Can you work these out from the model? Positions are in its coordinate system, mm. A direction names the side the tool comes from. Coordinates: 2 decimals unless noted, no trailing zeros. Order: outer loops, then holes, each group sorted by start corner. A loop starts at its lowest first (then second) coordinate and runs counter-clockwise, first axis right, second up. Notation, with made-up numbers: (80.25, 44.5) -> (86.25, 44.5) arc R17 cw to (86.25, 49.5) -> close; hole circle Ø11 at (67, 46.25). An arc over 180 degrees is marked (long way). Answer as a JSON object with one key per item and string values. Group by question number.
(1) I want a section at B-B, the plane z = -24.5. List the corners of the cut face in (x, y) for me.
(2) I need wall thicknesses on line 1 (X direction, y = 1, z = -24.5); line 2 (Z direction, x = -52.5, y = 2.45); line 3 (X direction, y = 1.9, z = -18). Which ranges of each line are inside material? Lowest first, please.
(3) I want a section at C-C, the plane y = 1.75. State how many separate pieces and enclosed holes the cut face has, plus the area to 3 significant figures.
(4) I want a section at A-A, the plane x = 52.5. List the corners of the cut face in (y, z) for me, plus the area to 3 significant figures.
(5) For pin 1 (5 mm diameter, centred on x = 30.5, y = 8, fed in from +Z); pin 2 (1.8 mm diameter, centred on x = 18, y = 7.5, fed in from +Z); pin 3 (1.3 mm diameter, centred on x = -12, y = 8, fed in from -Z); pin 4 (1 mm diameter, centred on x = 4, z = -8, fed in from +Y), each with a flat end and sliding along its axis, tell me the tip position at first contact or that it passes through.
(6) If we mould it in two halves opening along Z, with no side actions, what happens to faces 1 (the flat face through (15, 5, 18)), 2 (the flat face through (12, 5, 3)), 3 (the cylindrical face through (54.2, 1.48, -28.07))? For each: pulls with the +Z half, pulls with the -Z half, needs draft (parallel to the pull), parting line crosses it, or undercut.
(7) Which directions (+Z, -Z, +X, -X, +Y, -Y) give clear straight access to the entire face, cutting with the end or side of a thin tool? Please do faces 4 (the flat face through (52, 1, -13)), 5 (the flat face through (-31, 7, 21)), 6 (the flat face through (11, 6, 17)).
from build123d import *

# Parameters (mm, degrees)
BOSS_EXTRUDE1_DEPTH  = 3
M3_CLEARANCE_HOLE1_D = 3.4
M3_CLEARANCE_HOLE2_D = 3.4
EXTRUDE_THIN1_DEPTH  = 6
SKETCH9_W            = 1
SKETCH9_H            = 1.2
CHAMFER1_SIZE        = 1
SKETCH11_W           = 22
SKETCH11_H           = 3
CUT_EXTRUDE1_DEPTH   = 6
SKETCH12_W           = 6
SKETCH12_H           = 30
BOSS_EXTRUDE3_DEPTH  = 11
CHAMFER2_SIZE        = 6
CHAMFER3_SIZE        = 11


# Some blends are built 0.0001 mm under size
with BuildPart() as part:
    # Sketch1 → Boss-Extrude1 (new body)
    with BuildSketch(Plane(origin=(0, 0, 0), x_dir=(1, 0, 0), z_dir=(0, 1, 0))):
        Polygon((-57.5, 33), (-57.5, 13), (-47.5, 13), (-47.5, -33), (47.5, -33), (47.5, 13), (57.5, 13), (57.5, 33), align=None)
    extrude(amount=BOSS_EXTRUDE1_DEPTH)

    # M3 Clearance Hole1 (through all)
    with Locations(Plane(origin=(0, 3, 0), x_dir=(1, 0, 0), z_dir=(0, 1, 0))):
        with Locations((-52.5, 28), (-52.5, 18), (52.5, 28), (52.5, 18)):
            Hole(M3_CLEARANCE_HOLE1_D / 2)

    # M3 Clearance Hole2 (through all)
    with Locations(Plane(origin=(0, 3, 0), x_dir=(1, 0, 0), z_dir=(0, 1, 0))):
        with Locations((-19, 24.5), (-19, -24.5), (39, -24.5), (39, 24.5)):
            Hole(M3_CLEARANCE_HOLE2_D / 2)

    # Sketch8 → Extrude-Thin1 (add)
    with BuildSketch(Plane(origin=(0, 3, 0), x_dir=(1, 0, 0), z_dir=(0, 1, 0))):
        Polygon((-12, 8.5), (-12, -15), (12, -15), (12, 8.5), (15, 8.5), (15, -18), (-15, -18), (-15, 8.5), align=None)
    extrude(amount=EXTRUDE_THIN1_DEPTH)

    # Cut-Sweep1: sweep along a path in Sketch10
    with BuildLine(Plane(origin=(0, 7.6, 0), x_dir=(1, 0, 0), z_dir=(0, 1, 0))) as cut_sweep1_path:
        Line((12, 8.5), (12, -15))
        Line((12, -15), (-12, -15))
        Line((-12, -15), (-12, 8.5))
    # Sketch9 → Cut-Sweep1 (sweep, cut)
    with BuildSketch(Plane(origin=(0, 0, -8.5), x_dir=(-1, 0, 0), z_dir=(0, 0, -1))):
        with Locations((-12.5, 7.6)):
            Rectangle(SKETCH9_W, SKETCH9_H)
    sweep(path=cut_sweep1_path.line, transition=Transition.RIGHT, mode=Mode.SUBTRACT)

    # Chamfer1
    # the kernel refuses this chamfer: 1 mm, written as the material it takes off along each edge
    with BuildSketch(Plane(origin=(-12, 8.2, 15), x_dir=(-0.9996219169112968, -0.0274958766105856, 0), z_dir=(0, 0, -1))) as chamfer1_piece_1_section:
        Polygon((CHAMFER1_SIZE * 0.999621916911, CHAMFER1_SIZE * 0.0274958766106), (-CHAMFER1_SIZE * 0.0274958766106, CHAMFER1_SIZE * 0.999621916911), (0, 0), align=None)
    chamfer1_piece_1 = extrude(amount=26.071682988, mode=Mode.PRIVATE)
    chamfer1_piece_1 = split(chamfer1_piece_1, bisect_by=Plane(origin=(-13, 8.530404154, 1.964158506), z_dir=(1, 0, 0)), keep=Keep.TOP, mode=Mode.PRIVATE)
    add(chamfer1_piece_1, mode=Mode.SUBTRACT)
    with BuildSketch(Plane(origin=(12, 8.2, 15), x_dir=(0, -0.0274958766105856, 0.9996219169112968), z_dir=(-1, 0, 0))) as chamfer1_piece_2_section:
        Polygon((CHAMFER1_SIZE * 0.999621916911, CHAMFER1_SIZE * 0.0274958766106), (-CHAMFER1_SIZE * 0.0274958766106, CHAMFER1_SIZE * 0.999621916911), (0, 0), align=None)
    chamfer1_piece_2 = extrude(amount=24, mode=Mode.PRIVATE)
    chamfer1_piece_2 = split(chamfer1_piece_2, bisect_by=Plane(origin=(0, 8.530404154, 16), z_dir=(0, 0, -1)), keep=Keep.TOP, mode=Mode.PRIVATE)
    add(chamfer1_piece_2, mode=Mode.SUBTRACT)
    with BuildSketch(Plane(origin=(12, 8.2, -11.071682988), x_dir=(0.9996219169112968, -0.027495876610585647, 0), z_dir=(0, 0, 1))) as chamfer1_piece_3_section:
        Polygon((CHAMFER1_SIZE * 0.999621916911, CHAMFER1_SIZE * 0.0274958766106), (-CHAMFER1_SIZE * 0.0274958766106, CHAMFER1_SIZE * 0.999621916911), (0, 0), align=None)
    chamfer1_piece_3 = extrude(amount=26.071682988, mode=Mode.PRIVATE)
    chamfer1_piece_3 = split(chamfer1_piece_3, bisect_by=Plane(origin=(13, 8.530404154, 1.964158506), z_dir=(-1, 0, 0)), keep=Keep.TOP, mode=Mode.PRIVATE)
    add(chamfer1_piece_3, mode=Mode.SUBTRACT)
    with BuildSketch(Plane(origin=(-12, 8.2, 17.571682988), x_dir=(-0.9996219169112968, -0.027495876610585647, 0), z_dir=(0, 0, -1))) as chamfer1_piece_4a_section:
        Polygon((CHAMFER1_SIZE * 0.999621916911, CHAMFER1_SIZE * 0.0274958766106), (-CHAMFER1_SIZE * 0.0274958766106, CHAMFER1_SIZE * 0.999621916911), (0, 0), align=None)
    chamfer1_piece_4a = extrude(amount=28.643365976, mode=Mode.PRIVATE)
    chamfer1_piece_4a = split(chamfer1_piece_4a, bisect_by=Plane(origin=(-13, 8.530404154, 15.5), z_dir=(1, 0, 0)), keep=Keep.TOP, mode=Mode.PRIVATE)
    chamfer1_piece_4a = split(chamfer1_piece_4a, bisect_by=Plane(origin=(-12.328634334, 8.530404154, 16), z_dir=(0, 0, -1)), keep=Keep.TOP, mode=Mode.PRIVATE)
    chamfer1_piece_4a = split(chamfer1_piece_4a, bisect_by=Plane(origin=(-12.328634334, 8.530404154, 15), z_dir=(0, 0, 1)), keep=Keep.TOP, mode=Mode.PRIVATE)
    with BuildSketch(Plane(origin=(12, 8.2, 15), x_dir=(0, -0.0274958766105856, 0.9996219169112968), z_dir=(-1, 0, 0))) as chamfer1_piece_4b_section:
        Polygon((CHAMFER1_SIZE * 0.999621916911, CHAMFER1_SIZE * 0.0274958766106), (-CHAMFER1_SIZE * 0.0274958766106, CHAMFER1_SIZE * 0.999621916911), (0, 0), align=None)
    chamfer1_piece_4b = extrude(amount=26.571682988, mode=Mode.PRIVATE)
    chamfer1_piece_4b = split(chamfer1_piece_4b, bisect_by=Plane(origin=(-13, 8.530404154, 15.328634334), z_dir=(1, 0, 0)), keep=Keep.TOP, mode=Mode.PRIVATE)
    chamfer1_piece_4b = split(chamfer1_piece_4b, bisect_by=Plane(origin=(-12.5, 8.530404154, 16), z_dir=(0, 0, -1)), keep=Keep.TOP, mode=Mode.PRIVATE)
    chamfer1_piece_4b = split(chamfer1_piece_4b, bisect_by=Plane(origin=(-12, 8.530404154, 15.328634334), z_dir=(-1, 0, 0)), keep=Keep.TOP, mode=Mode.PRIVATE)
    chamfer1_piece_4 = chamfer1_piece_4a & chamfer1_piece_4b
    add(chamfer1_piece_4, mode=Mode.SUBTRACT)
    with BuildSketch(Plane(origin=(12, 8.2, -11.071682988), x_dir=(0.9996219169112968, -0.027495876610585647, 0), z_dir=(0, 0, 1))) as chamfer1_piece_5a_section:
        Polygon((CHAMFER1_SIZE * 0.999621916911, CHAMFER1_SIZE * 0.0274958766106), (-CHAMFER1_SIZE * 0.0274958766106, CHAMFER1_SIZE * 0.999621916911), (0, 0), align=None)
    chamfer1_piece_5a = extrude(amount=28.643365976, mode=Mode.PRIVATE)
    chamfer1_piece_5a = split(chamfer1_piece_5a, bisect_by=Plane(origin=(13, 8.530404154, 15.5), z_dir=(-1, 0, 0)), keep=Keep.TOP, mode=Mode.PRIVATE)
    chamfer1_piece_5a = split(chamfer1_piece_5a, bisect_by=Plane(origin=(12.328634334, 8.530404154, 16), z_dir=(0, 0, -1)), keep=Keep.TOP, mode=Mode.PRIVATE)
    chamfer1_piece_5a = split(chamfer1_piece_5a, bisect_by=Plane(origin=(12.328634334, 8.530404154, 15), z_dir=(0, 0, 1)), keep=Keep.TOP, mode=Mode.PRIVATE)
    with BuildSketch(Plane(origin=(14.571682988, 8.2, 15), x_dir=(0, -0.0274958766105856, 0.9996219169112968), z_dir=(-1, 0, 0))) as chamfer1_piece_5b_section:
        Polygon((CHAMFER1_SIZE * 0.999621916911, CHAMFER1_SIZE * 0.0274958766106), (-CHAMFER1_SIZE * 0.0274958766106, CHAMFER1_SIZE * 0.999621916911), (0, 0), align=None)
    chamfer1_piece_5b = extrude(amount=26.571682988, mode=Mode.PRIVATE)
    chamfer1_piece_5b = split(chamfer1_piece_5b, bisect_by=Plane(origin=(13, 8.530404154, 15.328634334), z_dir=(-1, 0, 0)), keep=Keep.TOP, mode=Mode.PRIVATE)
    chamfer1_piece_5b = split(chamfer1_piece_5b, bisect_by=Plane(origin=(12.5, 8.530404154, 16), z_dir=(0, 0, -1)), keep=Keep.TOP, mode=Mode.PRIVATE)
    chamfer1_piece_5b = split(chamfer1_piece_5b, bisect_by=Plane(origin=(12, 8.530404154, 15.328634334), z_dir=(1, 0, 0)), keep=Keep.TOP, mode=Mode.PRIVATE)
    chamfer1_piece_5 = chamfer1_piece_5a & chamfer1_piece_5b
    add(chamfer1_piece_5, mode=Mode.SUBTRACT)

    # Sketch11 → Cut-Extrude1 (cut)
    with BuildSketch(Plane(origin=(0, 9, 0), x_dir=(1, 0, 0), z_dir=(0, 1, 0))):
        with Locations((0, -16.5)):
            Rectangle(SKETCH11_W, SKETCH11_H)
    extrude(amount=-CUT_EXTRUDE1_DEPTH, mode=Mode.SUBTRACT)

    # Sketch12 → Boss-Extrude3 (add)
    with BuildSketch(Plane(origin=(0, 3, 0), x_dir=(1, 0, 0), z_dir=(0, 1, 0))):
        with Locations((-27, -6)):
            Rectangle(SKETCH12_W, SKETCH12_H)
        with Locations((27, -6)):
            Rectangle(SKETCH12_W, SKETCH12_H)
    extrude(amount=BOSS_EXTRUDE3_DEPTH)

    # Chamfer2
    chamfer2_edges = [part.edges().sort_by_distance(p)[0] for p in [
        (15, 3, 4.75),
        (-15, 3, 4.75),
    ]]
    chamfer(chamfer2_edges, length=CHAMFER2_SIZE - 0.0001)  # a hair under: the kernel refuses the full size

    # Chamfer3
    chamfer3_edges = [part.edges().sort_by_distance(p)[0] for p in [
        (30, 3, 6),
        (-30, 3, 6),
    ]]
    chamfer(chamfer3_edges, length=CHAMFER3_SIZE - 0.0001)  # a hair under: the kernel refuses the full size


solid = part.part
Computed values:
{
 "1": {"outline": "(-57.5, 0) -> (-20.7, 0) -> (-20.7, 3) -> (-57.5, 3) -> close; (-17.3, 0) -> (37.3, 0) -> (37.3, 3) -> (-17.3, 3) -> close; (40.7, 0) -> (57.5, 0) -> (57.5, 3) -> (40.7, 3) -> close"},
 "2": {"line 1": "x = -57.5 to -20.7, -17.3 to 37.3, 40.7 to 57.5", "line 2": "z = -33 to -29.7, -26.3 to -19.7, -16.3 to -13", "line 3": "x = -57.5 to -54.2, -50.8 to 50.8, 54.2 to 57.5"},
 "3": {"separate pieces": "1", "enclosed holes": "8", "area": "6,600 mm2"},
 "4": {"outline": "(0, -33) -> (3, -33) -> (3, -29.7) -> (0, -29.7) -> close; (0, -26.3) -> (3, -26.3) -> (3, -19.7) -> (0, -19.7) -> close; (0, -16.3) -> (3, -16.3) -> (3, -13) -> (0, -13) -> close", "area": "39.6 mm2"},
 "5": {"pin 1": "stops at z = 21", "pin 2": "passes through", "pin 3": "stops at z = 15.55", "pin 4": "stops at y = 3"},
 "6": {"face 1": "pulls with the +Z half", "face 2": "needs draft", "face 3": "undercut"},
 "7": {"face 4": "+Z, +X, +Y, -Y", "face 5": "+Z, +X, -X, +Y", "face 6": "+Z, -Z, +Y"}
}
